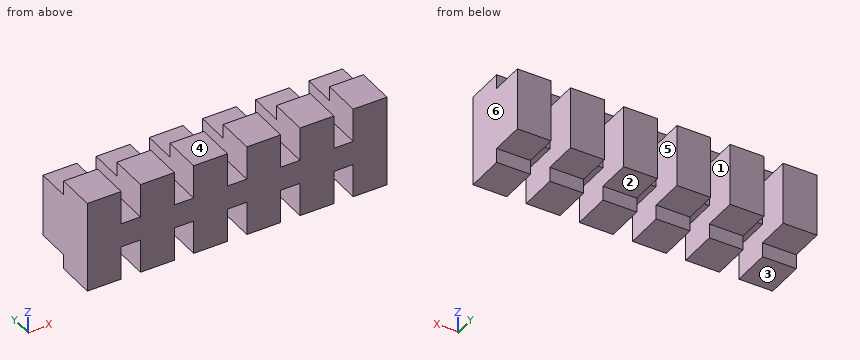
from build123d import *

# Parameters (mm, degrees)
BOSS_EXTRUDE1_DEPTH = 8
BOSS_EXTRUDE2_DEPTH = 7


with BuildPart() as part:
    # Sketch1 → Boss-Extrude1 (new body)
    with BuildSketch(Plane(origin=(0, 0, 0), x_dir=(1, 0, 0), z_dir=(0, 1, 0))):
        Polygon((-13, 2.5), (-13, 9.5), (-20, 9.5), (-20, 2.5), (-24, 2.5), (-24, 9.5), (-31, 9.5), (-31, -9.5), (-24, -9.5), (-24, -2.5), (-20, -2.5), (-20, -9.5), (-13, -9.5), (-13, -2.5), (-9, -2.5), (-9, -9.5), (-2, -9.5), (-2, -2.5), (2, -2.5), (2, -9.5), (9, -9.5), (9, -2.5), (13, -2.5), (13, -9.5), (20, -9.5), (20, -2.5), (24, -2.5), (24, -9.5), (31, -9.5), (31, 9.5), (24, 9.5), (24, 2.5), (20, 2.5), (20, 9.5), (13, 9.5), (13, 2.5), (9, 2.5), (9, 9.5), (2, 9.5), (2, 2.5), (-2, 2.5), (-2, 9.5), (-9, 9.5), (-9, 2.5), align=None)
    extrude(amount=-BOSS_EXTRUDE1_DEPTH)

    # Sketch2 → Boss-Extrude2 (add)
    with BuildSketch(Plane(origin=(0, 0, 0), x_dir=(1, 0, 0), z_dir=(0, 1, 0))):
        Polygon((-31, 6.5), (-24, 6.5), (-24, 2.5), (-24, -2.5), (-24, -6.5), (-31, -6.5), align=None)
        Polygon((-20, 6.5), (-13, 6.5), (-13, 2.5), (-13, -2.5), (-13, -6.5), (-20, -6.5), (-20, -2.5), (-20, 2.5), align=None)
        Polygon((-9, 6.5), (-2, 6.5), (-2, 2.5), (-2, -2.5), (-2, -6.5), (-9, -6.5), (-9, -2.5), (-9, 2.5), align=None)
        Polygon((2, 6.5), (9, 6.5), (9, 2.5), (9, -2.5), (9, -6.5), (2, -6.5), (2, -2.5), (2, 2.5), align=None)
        Polygon((13, 6.5), (20, 6.5), (20, 2.5), (20, -2.5), (20, -6.5), (13, -6.5), (13, -2.5), (13, 2.5), align=None)
        Polygon((24, 6.5), (31, 6.5), (31, -6.5), (24, -6.5), (24, -2.5), (24, 2.5), align=None)
    extrude(amount=BOSS_EXTRUDE2_DEPTH)


solid = part.part
Here's how the part is built. I have some questions about the finished solid (model axes, mm). Face numbers are marked on the shaded views. A direction names the side the tool comes from. Give positions to 0.01 mm unless a question says otherwise; leave off trailing zeros. Order: outer loops, then holes, each group sorted by start corner. A loop starts at its lowest first (then second) coordinate and runs counter-clockwise, first axis right, second up. Notation, with made-up numbers: (-20.75, 78) -> (36.25, 78) arc R24 cw to (36.25, 91) -> close; hole circle Ø8 at (68.25, 27.25). An arc over 180 degrees is marked (long way). Use a Markdown table: item, result. Add a question column.
Item 1: Will these pins go through, and if not, where does the flat tip stop? pin 1 (3.5 mm diameter, centred on x = -26.5, y = 2, fed in from -Z); pin 2 (2 mm diameter, centred on x = 22, z = 0.5, fed in from +Y); pin 3 (3.5 mm diameter, centred on x = -26, y = 3.5, fed in from +Z).
Item 2: For the marked faces 1, 2 and 3, which set-ups out of +Z, -Z, +X, -X, +Y, -Y let a thin tool reach every point of the face, with its end or its side?
Item 3: Imagine slicing it at D-D on x = 27. Please give me the cut outline in (y, z).
Item 4: Imagine slicing it at C-C on z = -1. Please give me the cut outline in (x, y).
Item 5: If we mould it in two halves opening along X, with no side actions, what happens to the marked faces 4, 5 and 6? For each: pulls with the +X half, pulls with the -X half, needs draft (parallel to the pull), parting line crosses it, or undercut.
Item 6: Imagine slicing it at B-B on y = 1.25. Please give me the cut outline in (x, z).
Item 7: I need wall thicknesses on line 1 (X direction, y = 5.5, z = -4.75); line 2 (Z direction, x = -27.5, y = 0.5); line 3 (Y direction, x = 28, z = 8.5). Which ranges of each line are inside material? Lowest first, please.
Item 8: Imagine slicing it at A-A on z = -8.25. Please give me the cut outline in (x, y).
Data:
| question | item | result |
|---|---|---|
| 1 | pin 1 | stops at z = -6.5 |
| 1 | pin 2 | stops at y = 0 |
| 1 | pin 3 | stops at z = 6.5 |
| 2 | face 1 | +Y |
| 2 | face 2 | -Z, +X, -X, +Y |
| 2 | face 3 | -Z, +X, -X, +Y, -Y |
| 3 | outline | (-8, -9.5) -> (0, -9.5) -> (0, -6.5) -> (7, -6.5) -> (7, 6.5) -> (0, 6.5) -> (0, 9.5) -> (-8, 9.5) -> close |
| 4 | outline | (-31, -8) -> (31, -8) -> (31, 7) -> (24, 7) -> (24, 0) -> (20, 0) -> (20, 7) -> (13, 7) -> (13, 0) -> (9, 0) -> (9, 7) -> (2, 7) -> (2, 0) -> (-2, 0) -> (-2, 7) -> (-9, 7) -> (-9, 0) -> (-13, 0) -> (-13, 7) -> (-20, 7) -> (-20, 0) -> (-24, 0) -> (-24, 7) -> (-31, 7) -> close |
| 5 | face 4 | needs draft |
| 5 | face 5 | undercut |
| 5 | face 6 | pulls with the +X half |
| 6 | outline | (-31, -6.5) -> (-24, -6.5) -> (-24, 6.5) -> (-31, 6.5) -> close; (-20, -6.5) -> (-13, -6.5) -> (-13, 6.5) -> (-20, 6.5) -> close; (-9, -6.5) -> (-2, -6.5) -> (-2, 6.5) -> (-9, 6.5) -> close; (2, -6.5) -> (9, -6.5) -> (9, 6.5) -> (2, 6.5) -> close; (13, -6.5) -> (20, -6.5) -> (20, 6.5) -> (13, 6.5) -> close; (24, -6.5) -> (31, -6.5) -> (31, 6.5) -> (24, 6.5) -> close |
| 7 | line 1 | x = -31 to -24, -20 to -13, -9 to -2, 2 to 9, 13 to 20, 24 to 31 |
| 7 | line 2 | z = -6.5 to 6.5 |
| 7 | line 3 | y = -8 to 0 |
| 8 | outline | (-31, -8) -> (-24, -8) -> (-24, 0) -> (-31, 0) -> close; (-20, -8) -> (-13, -8) -> (-13, 0) -> (-20, 0) -> close; (-9, -8) -> (-2, -8) -> (-2, 0) -> (-9, 0) -> close; (2, -8) -> (9, -8) -> (9, 0) -> (2, 0) -> close; (13, -8) -> (20, -8) -> (20, 0) -> (13, 0) -> close; (24, -8) -> (31, -8) -> (31, 0) -> (24, 0) -> close |
